Check sheet for the drawn part. Datum: minimum x, y, z corner. Units: mm. A direction names the side the tool comes from. Round coordinates to 2 decimals unless told otherwise and drop trailing zeros. Write each loop counter-clockwise with the first axis right and the second up, starting at its lowest first coordinate (ties: lowest second). Pieces come first, ordered by that corner, then holes.
Item 1: Cross-section at A-A on x = 21. Enter the section's corners in (y, z) (1 decimal), plus the area to 3 significant figures.
Item 2: Cross-section at C-C on y = 22. Enter the section's corners in (x, z) (1 decimal), plus the area to 3 significant figures.
Item 3: Tool access check on the marked faces 4 and 5. Record the directions out of +Z, -Z, +X, -X, +Y, -Y that give a thin tool (end or side, any length) a straight path to the whole face; none if there is none.
Item 4: Material ranges on line 1 (Y direction, x = 52.5, z = 33); line 2 (X direction, y = 29.5, z = 16); line 3 (X direction, y = 47.5, z = 23.5), recorded low to high.
Item 5: Cross-section at B-B on z = 7. Enter the section's corners in (x, y), plus the area to 3 significant figures.
Item 6: Go/stop test with flat-tipped pins: pin 1 Ø18.5 at (x, z) = (20.5, 40.5) entering from +Y; pin 2 Ø14 at (x, y) = (25.5, 110.5) entering from -Z (3 decimals); pin 3 Ø4 at (y, z) = (82, 47.5) entering from -X (1 decimal). Record where each tip stops, or that it passes through.
Item 7: Release check for a two-part mould opening along Z. For the marked faces 1, 2 and 3 record: +Z half, -Z half, draft (parallel to the pull), parting line (faces both ways), or undercut.
Item 8: Cross-section at D-D on x = 32.5. Enter the section's corners in (y, z) (1 decimal).
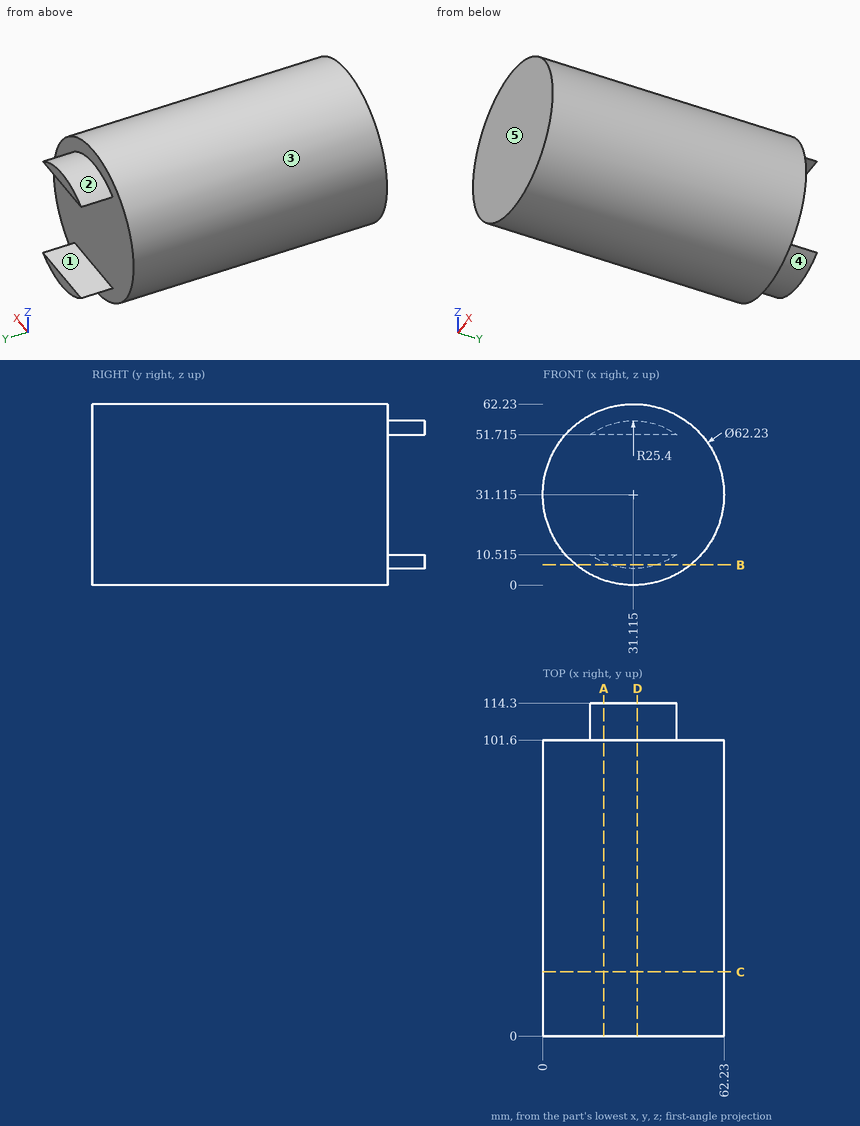
Response values:
1. outline: (0, 1.7) - (101.6, 1.7) - (101.6, 7.8) - (114.3, 7.8) - (114.3, 10.5) - (101.6, 10.5) - (101.6, 51.7) - (114.3, 51.7) - (114.3, 54.4) - (101.6, 54.4) - (101.6, 60.5) - (0, 60.5) - close
1. area: 6,050 mm2
2. outline: circle Ø62.2 at (31.1, 31.1)
2. area: 3,040 mm2
3. face 4: -Z, +Y
3. face 5: +Z, -Z, +X, -X, -Y
4. line 1: y = 0 to 101.6
4. line 2: x = 3.92 to 58.31
4. line 3: x = 0.95 to 61.28
5. outline: (11.45, 0) - (50.78, 0) - (50.78, 101.6) - (39.09, 101.6) - (39.09, 114.3) - (23.14, 114.3) - (23.14, 101.6) - (11.45, 101.6) - close
5. area: 4,200 mm2
6. pin 1: stops at y = 101.6
6. pin 2: stops at z = 5.715
6. pin 3: stops at x = 3.5
7. face 1: undercut
7. face 2: +Z half
7. face 3: parting line
8. outline: (0, 0) - (101.6, 0) - (101.6, 5.8) - (114.3, 5.8) - (114.3, 10.5) - (101.6, 10.5) - (101.6, 51.7) - (114.3, 51.7) - (114.3, 56.5) - (101.6, 56.5) - (101.6, 62.2) - (0, 62.2) - close
